The listing builds one solid part. Answer for the finished solid, in the listing's coordinates (mm). A direction names the side the tool comes from. Round coordinates to 2 decimals unless told otherwise and drop trailing zeros. Loops run counter-clockwise (first coordinate to the right, second up) from the corner with the lowest first, then second, coordinate; pieces in that order, holes last. Notation, with made-up numbers: (36, 82.5) - (68, 82.5) arc R27 ccw to (68, 112.5) - close; hole circle Ø2 at (-13.5, 84). An arc over 180 degrees is marked (long way). Write item = value, one per line. Start each with the question number.
1) Given pin 1 Ø11.5 at (x, y) = (0, 0) entering from -Z (3 decimals); pin 2 Ø17 at (y, z) = (-19.5, 19.5) entering from +X; pin 3 Ø5 at (x, y) = (-1.5, 18.5) entering from +Z (3 decimals); pin 4 Ø8 at (x, z) = (-8.5, 16.5) entering from +Y, each flat-ended and moving along its own axis, determine where each tip first touches the part or whether it passes through.
2) For a pull along X with two mould halves and no side action, classify faces 4 (the cylindrical face through (-1.087, -4.897, 0.044)), 5 (the flat face through (12, 0, -3.175)), 6 (the flat face through (-31.75, -11, 11)) as released by +X, released by -X, zero draft, split by the parting line, or undercut.
3) Section C-C, the plane z = 1 is taken. Determine the outline of the cut face in (x, y).
4) Section D-D, the plane y = -18 is taken. Determine the outline of the cut face in (x, z) (3 decimals), and give its area (3 significant figures).
5) A tool of negligible diameter and unlimited length cuts with its end or side. For faces 1 (the flat face through (31.75, -18, 19)), 2 (the flat face through (0, -18, 34.925)), 3 (the flat face through (0, -10.16, 19)), from which of +Z, -Z, +X, -X, +Y, -Y can it reach the whole face along a straight path? Write none if from no direction.
6) Straight lines are drawn through the part: line 1 along Y through (x, z) = (0, 2); line 2 along Y through (x, z) = (29, 26); line 3 along Z through (x, y) = (-4, 14.5) (3 decimals). For each, find the intervals that lie inside material, in ascending order.
7) Section B-B, the plane x = 0 is taken. Determine the outline of the cut face in (y, z) (1 decimal).
Autodesk Inventor part; units mm, degrees
ref_plane "YZ Plane" through (0, 0, 0) normal (1, 0, 0) x (0, 1, 0)
ref_plane "XZ Plane" through (0, 0, 0) normal (0, 1, 0) x (-1, 0, 0)
ref_plane "XY Plane" through (0, 0, 0) normal (0, 0, 1) x (1, 0, 0)
sketch "Sketch2" plane through (0, 0, 0) normal (0, 0, 1) x (1, 0, 0)
  line L0 (0, 0) -> (-31.75, 0) construction
  line L1 (-31.75, 0) -> (-31.75, -25.4)
  line L2 (-31.75, 0) -> (-31.75, 25.4)
  line L3 (-31.75, 25.4) -> (57.15, 25.4)
  line L4 (0, 0) -> (0, -25.4) construction
  line L5 (0, 0) -> (57.15, 0) construction
  line L6 (-31.75, -25.4) -> (57.15, -25.4)
  line L7 (57.15, 25.4) -> (57.15, -25.4)
  dimension "edgeToCenterOfPiston" = 31.75
  dimension "heiight" = 50.8
  dimension "width" = 88.9
  dimension "d7" = 88.9
  dimension "d8" = 88.9
extrude "Extrusion1" add sketch "Sketch2" along normal mid plane 6.35
sketch "Sketch3" plane through (0, 0, 3.175) normal (0, 0, 1) x (1, 0, 0)
  circle A0 centre (0, 0) radius 5.0165
  dimension "d11" = 10.033
extrude "Extrusion2" cut sketch "Sketch3" against normal through all
sketch "Sketch4" plane through (0, 0, 3.175) normal (0, 0, 1) x (1, 0, 0)
  line L0 (-31.75, 25.4) -> (-31.75, -25.4)
  line L1 (-31.75, -25.4) -> (31.75, -25.4)
  line L2 (31.75, -25.4) -> (31.75, -10.16)
  line L3 (31.75, -10.16) -> (-31.75, -10.16)
  line L4 (-31.75, -10.16) -> (-31.75, -25.4)
  point P0 (0, 0)
  dimension "d14" = 63.5
  dimension "d15" = 15.24
extrude "Extrusion3" add sketch "Sketch4" along normal blind 31.75
equation "\"d7\" = width"
equation "\"d8\" = width"
properties part number "Gripper Piston" material "Aluminum 6061"
Geometry check:
q1.pin_1 = -3.175
q1.pin_2 = 31.75
q1.pin_3 = 3.175
q1.pin_4 = -10.16
q2.face_4 = undercut
q2.face_5 = zero draft
q2.face_6 = released by -X
q3.outline = (-31.75, -25.4) - (57.15, -25.4) - (57.15, 25.4) - (-31.75, 25.4) - close; hole circle Ø10.03 at (0, 0)
q4.outline = (-31.75, -3.175) - (57.15, -3.175) - (57.15, 3.175) - (31.75, 3.175) - (31.75, 34.925) - (-31.75, 34.925) - close
q4.area = 2,580 mm2
q5.face_1 = +Z, +X, +Y, -Y
q5.face_2 = +Z, +X, -X, +Y, -Y
q5.face_3 = +Z, +X, -X, +Y
q6.line_1 = -25.4 to -5.02, 5.02 to 25.4
q6.line_2 = -25.4 to -10.16
q6.line_3 = -3.175 to 3.175
q7.outline = (-25.4, -3.2) - (-5, -3.2) - (-5, 3.2) - (-10.2, 3.2) - (-10.2, 34.9) - (-25.4, 34.9) - close; (5, -3.2) - (25.4, -3.2) - (25.4, 3.2) - (5, 3.2) - close
